Design review of the part built by this model. Coordinates are the model's own, in mm. A direction names the side the tool comes from. Round coordinates to 2 decimals unless told otherwise and drop trailing zeros. Loops run counter-clockwise (first coordinate to the right, second up) from the corner with the lowest first, then second, coordinate; pieces in that order, holes last. Notation, with made-up numbers: M 11,29 L 45,29 A24 ccw 45,54 Z; hole C 28.5,46 d8. An arc over 180 degrees is marked long. Use a Markdown table: item, result.
from build123d import *

# Parameters (mm, degrees)
BASE_EXTRUDE_DEPTH = 15


with BuildPart() as part:
    # Sketch1 → Base-Extrude (new, symmetric)
    with BuildSketch(Plane.XY):
        with BuildLine():
            Line((0, 2.08), (0, 2.5))
            ThreePointArc((0, 2.5), (-1.767766953, -1.767766953), (2.5, 0))
            ThreePointArc((2.5, 0), (1.680782105, 1.557766953), (0, 2.08))
        make_face()
        with BuildLine():
            Line((-2.08, 0), (-1.66, 0))
            ThreePointArc((-1.66, 0), (-1.173797257, 1.173797257), (0, 1.66))
            ThreePointArc((0, 1.66), (1.383797257, 1.260782105), (2.08, 0))
            ThreePointArc((2.08, 0), (0, -2.08), (-2.08, 0))
        make_face(mode=Mode.SUBTRACT)
    extrude(amount=BASE_EXTRUDE_DEPTH, both=True)


solid = part.part
1. Machinability: for faces 1 (the face through (-1.3, 1.3, -15)), 2 (the face through (0.05, -2.08, 0.21)), which of the approach directions +Z, -Z, +X, -X, +Y, -Y give a long, thin tool a straight path to every point of the face, cutting with its end or side? Answer none if there is none.
Check values:
| item | result |
|---|---|
| face 1 | -Z, +X, -X, +Y, -Y |
| face 2 | +Z, -Z |
2. Take a section at B-B on x = -1.4. Give the boundary of the cut face in (y, z), and give its area (3 significant figures).
Check values:
| item | result |
|---|---|
| outline | M -2.07,-15 L -1.54,-15 L -1.54,15 L -2.07,15 Z; M 0.89,-15 L 2.07,-15 L 2.07,15 L 0.89,15 Z |
| area | 51.4 mm² |
3. Take a section at A-A on z = -7.5. Give the boundary of the cut face in (x, y), and give its area (3 significant figures).
Check values:
| item | result |
|---|---|
| outline | M 0,2.08 L 0,2.5 A2.5 ccw long 2.5,0 A2.3 ccw Z; hole M -2.08,0 A2.08 ccw 2.08,0 A1.88 ccw 0,1.66 A1.66 ccw -1.66,0 Z |
| area | 7.14 mm² |
4. Take a section at C-C on y = 1.15. Give the boundary of the cut face in (x, z), and give its area (3 significant figures).
Check values:
| item | result |
|---|---|
| outline | M -2.22,-15 L -1.2,-15 L -1.2,15 L -2.22,15 Z; M 1.51,-15 L 2.06,-15 L 2.06,15 L 1.51,15 Z |
| area | 47.3 mm² |
5. Wall thickness on line 1 along Y through (x, z) = (-0.1, 6); line 2 along Y through (x, z) = (-0.2, -9); line 3 along X through (y, z) = (0.2, 13.75): over which ranges is each line inside the solid? List them lowest first. Write a range as from..to.
Check values:
| item | result |
|---|---|
| line 1 | y = -2.5..-2.08, 1.66..2.5 |
| line 2 | y = -2.49..-2.07, 1.65..2.49 |
| line 3 | x = -2.49..-1.65, 2.05..2.47 |
6. Insertion check: pin 1 (1.5 mm diameter, centred on y = -1, z = -9.5, fed in from +X). The pin has a flat end and moves straight along its axis. Give the tip position at first contact, or say it passes through.
Check values:
| item | result |
|---|---|
| pin 1 | stops at x = 2.49 |
7. The part is to be moulded in two halves that separate along Y. For faces 3 (the face through (-1.3, 1.3, 15)), 4 (the face through (-1.19, 1.16, 0.21)), 5 (the face through (1.7, 1.54, 0.21)), 6 (the face through (-1.825, -1.709, 0.21)), say which applies: pulls with the +Y half, pulls with the -Y half, needs draft (parallel to the pull), parting line crosses it, or undercut.
Check values:
| item | result |
|---|---|
| face 3 | needs draft |
| face 4 | undercut |
| face 5 | pulls with the +Y half |
| face 6 | parting line crosses it |
